Check sheet for the drawn part. Datum: minimum x, y, z corner. Units: mm. A direction names the side the tool comes from. Round coordinates to 2 decimals unless told otherwise and drop trailing zeros. Order: outer loops, then holes, each group sorted by start corner. A loop starts at its lowest first (then second) coordinate and runs counter-clockwise, first axis right, second up. Notation, with made-up numbers: (63, -28.5) -> (79, -28.5) arc R18 ccw to (79, -3.5) -> close; hole circle Ø11 at (87, -24.5). An arc over 180 degrees is marked (long way). Answer as a JSON object with one key per item and string values. Group by question number.
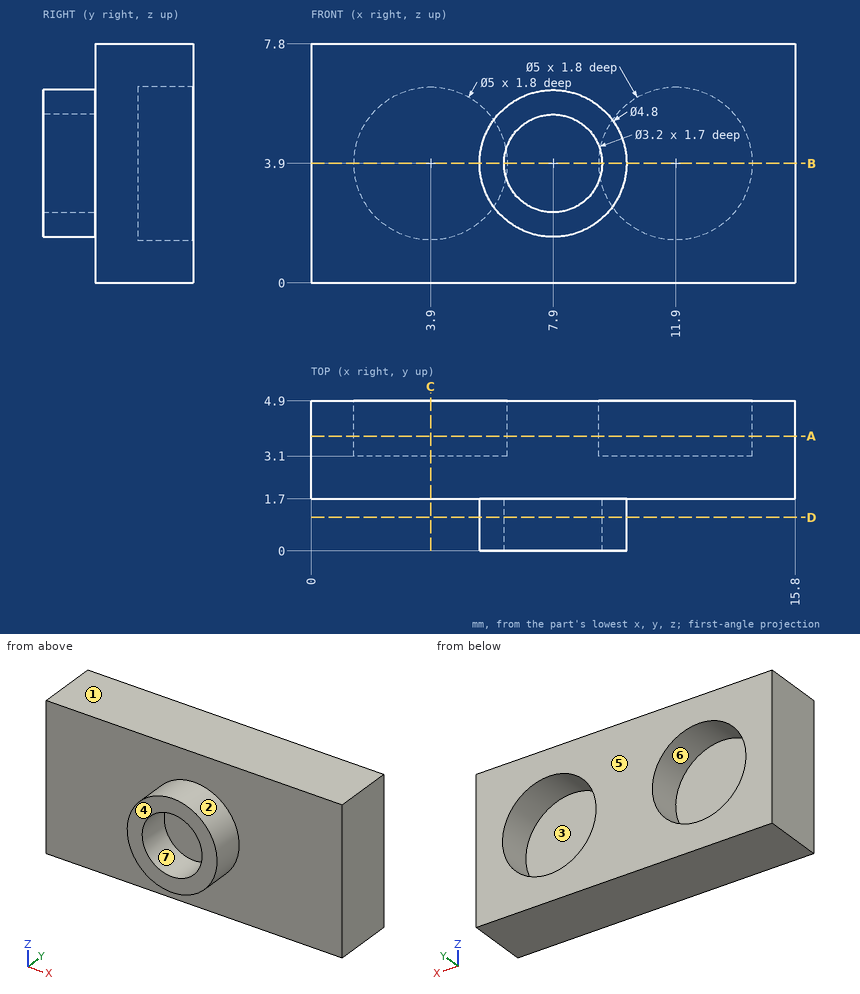
Item 1: Sectioned sample at D-D, the plane y = 1.1. Enter the section's corners in (x, z).
Item 2: Depth check by flat-ended pin: pin 1 Ø2 at (x, z) = (10, 6) entering from -Y; pin 2 Ø1.6 at (x, z) = (7.5, 4.5) entering from -Y; pin 3 Ø3 at (x, z) = (11.9, 3.9) entering from +Y. Enter the tip coordinate at first touch or a pass-through.
Item 3: Mould release check, pull along Z, two halves, no side actions. Record for the marked faces 1, 2, 3 and 4: pulls with the +Z half, pulls with the -Z half, needs draft (parallel to the pull), parting line crosses it, or undercut.
Item 4: Sectioned sample at B-B, the plane z = 3.9. Enter the section's corners in (x, y).
Item 5: Set-up check for the marked faces 5, 6 and 7: record each of +Z, -Z, +X, -X, +Y, -Y from which the full face is reachable in a straight line by a thin tool's end or side.
Item 6: Sectioned sample at C-C, the plane x = 3.9. Enter the section's corners in (y, z), then the cut area to 3 significant figures.
Item 7: Sectioned sample at A-A, the plane y = 3.75. Enter the section's corners in (x, z).
Item 8: Thickness scan on L1, parallel to X at y = 3.95, z = 3.9; L2, parallel to X at y = 0.85, z = 3.9; L3, parallel to X at y = 0.45, z = 3.5. Record the ranges inside material, lowest first.
Result:
{
 "1": {"outline": "circle Ø4.8 at (7.9, 3.9); hole circle Ø3.2 at (7.9, 3.9)"},
 "2": {"pin 1": "stops at y = 0", "pin 2": "stops at y = 1.7", "pin 3": "stops at y = 3.1"},
 "3": {"face 1": "pulls with the +Z half", "face 2": "parting line crosses it", "face 3": "undercut", "face 4": "needs draft"},
 "4": {"outline": "(0, 1.7) -> (5.5, 1.7) -> (5.5, 0) -> (6.3, 0) -> (6.3, 1.7) -> (9.5, 1.7) -> (9.5, 0) -> (10.3, 0) -> (10.3, 1.7) -> (15.8, 1.7) -> (15.8, 4.9) -> (14.4, 4.9) -> (14.4, 3.1) -> (9.4, 3.1) -> (9.4, 4.9) -> (6.4, 4.9) -> (6.4, 3.1) -> (1.4, 3.1) -> (1.4, 4.9) -> (0, 4.9) -> close"},
 "5": {"face 5": "+Z, -Z, +X, -X, +Y", "face 6": "+Y", "face 7": "-Y"},
 "6": {"outline": "(1.7, 0) -> (4.9, 0) -> (4.9, 1.4) -> (3.1, 1.4) -> (3.1, 6.4) -> (4.9, 6.4) -> (4.9, 7.8) -> (1.7, 7.8) -> close", "area": "16.0 mm2"},
 "7": {"outline": "(0, 0) -> (15.8, 0) -> (15.8, 7.8) -> (0, 7.8) -> close; hole circle Ø5 at (3.9, 3.9); hole circle Ø5 at (11.9, 3.9)"},
 "8": {"L1": "x = 0 to 1.4, 6.4 to 9.4, 14.4 to 15.8", "L2": "x = 5.5 to 6.3, 9.5 to 10.3", "L3": "x = 5.53 to 6.35, 9.45 to 10.27"}
}
